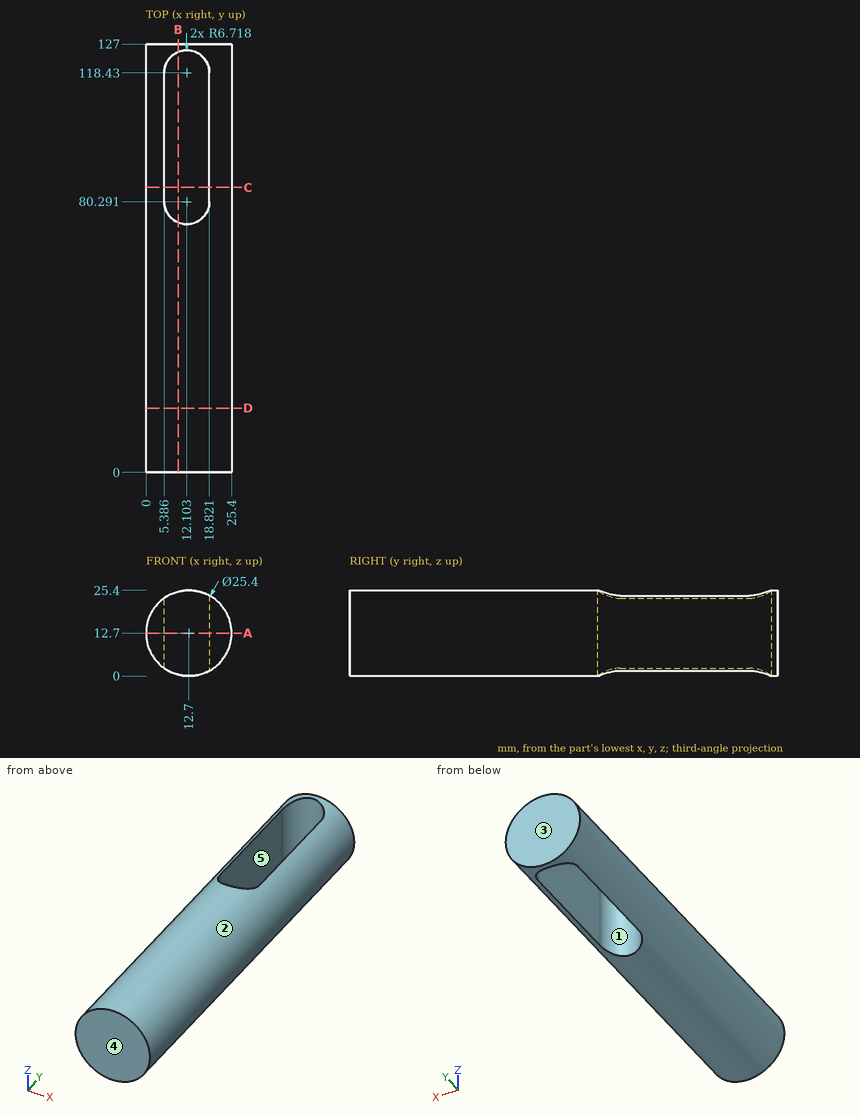
Geometry check sheet. Reference: drawing and pictorial views, mm from the part's lowest x, y, z. A direction names the side the tool comes from. Round coordinates to 2 decimals unless told otherwise and drop trailing zeros. Loops run counter-clockwise (first coordinate to the right, second up) from the corner with the lowest first, then second, coordinate; pieces in that order, holes last. Notation, with made-up numbers: M 81,63 L 129,63 A20 cw 129,72 Z; hole C -29.75,-26.75 d5. An arc over 180 degrees is marked long. Return JSON: item names as keys, results as strings. Group by question number.
(1) Section check C-C, the plane y = 84.5. Enter the section's corners in (x, z) (1 decimal).
(2) Scan lines: line 1 along X through (y, z) = (91.5, 17.5) (1 decimal); line 2 along X through (y, z) = (82.5, 2.75) (1 decimal); line 3 along Y through (x, z) = (17.5, 11). Record each from-to range of solid material in increasing order. Write a range as [from, to].
(3) Go/stop test with flat-tipped pins: pin 1 (5 mm diameter, centred on y = 97.5, z = 6.5, fed in from +X); pin 2 (1.5 mm diameter, centred on x = 10, y = 62, fed in from -Z); pin 3 (12 mm diameter, centred on y = 66.5, z = 3.5, fed in from +X). Record where each tip stops, or that it passes through.
(4) Section check D-D, the plane y = 19. Enter the section's corners in (x, z).
(5) Set-up check for the marked faces 1 and 2: record each of +Z, -Z, +X, -X, +Y, -Y from which the full face is reachable in a straight line by a thin tool's end or side.
(6) Section check B-B, the plane x = 9.5. Enter the section's corners in (y, z).
(7) Section check A-A, the plane z = 12.7. Enter the section's corners in (x, y) (1 decimal), and give its area (3 significant figures).
(8) Mould release check, pull along Y, two halves, no side actions. Record for the marked faces 3, 4 and 5: pulls with the +Y half, pulls with the -Y half, needs draft (parallel to the pull), parting line crosses it, or undercut.
Data:
{
 "1": {"outline": "M 5.4,2.3 L 5.4,23.1 A12.7 ccw Z; M 18.8,1.6 A12.7 ccw 18.8,23.8 Z"},
 "2": {"line 1": "[0.9, 5.4], [18.8, 24.5]", "line 2": "[4.8, 5.4], [18.8, 20.6]", "line 3": "[0, 76.29], [122.43, 127]"},
 "3": {"pin 1": "x = 24.85", "pin 2": "z = 0.15", "pin 3": "x = 24.99"},
 "4": {"outline": "C 12.7,12.7 d25.4"},
 "5": {"face 1": "+Z, -Z", "face 2": "+Y, -Y"},
 "6": {"outline": "M 0,0.41 L 74.1,0.41 L 74.1,24.99 L 0,24.99 Z; M 124.62,0.41 L 127,0.41 L 127,24.99 L 124.62,24.99 Z"},
 "7": {"outline": "M 0,0 L 25.4,0 L 25.4,127 L 0,127 Z; hole M 5.4,80.3 A6.7 ccw 18.8,80.3 L 18.8,118.4 A6.7 ccw 5.4,118.4 Z", "area": "2,570 mm²"},
 "8": {"face 3": "pulls with the +Y half", "face 4": "pulls with the -Y half", "face 5": "undercut"}
}
